```python
from build123d import *

# Parameters (mm, degrees)
F1_DEPTH = 10
F2_D     = 5.3
F4_D     = 4.2
F4_DEPTH = 10.4
F4_TIP   = 1.2618073


with BuildPart() as f1:
    # F0 (on Front) → F1 (new body)
    with BuildSketch(Plane.XZ):
        Polygon((35, -20), (35, 0), (35, 20), (-35, 20), (-35, -20), (-5.4585481157, -20), (-9.5, -27), (0, -27), (9.5, -27), (5.4585481157, -20), align=None)
    extrude(amount=-F1_DEPTH)

    # F2 (through all)
    with Locations(Plane.XZ):
        with Locations((0, 0)):
            Hole(F2_D / 2)

    # F4
    with Locations(Plane(origin=(0, 0, -20), x_dir=(1, 0, 0), z_dir=(0, 0, -1))):
        with Locations((-20, -5), (20, -5)):
            Hole(F4_D / 2, depth=F4_DEPTH)
            with Locations((0, 0, -(F4_DEPTH + F4_TIP / 2))):  # 118° drill point
                Cone(0, F4_D / 2, F4_TIP, mode=Mode.SUBTRACT)


solid = f1.part
```
Build history of the part. All positions in model axes, mm. A direction names the side the tool comes from. Round coordinates to 2 decimals unless told otherwise and drop trailing zeros. Loops run counter-clockwise (first coordinate to the right, second up) from the corner with the lowest first, then second, coordinate; pieces in that order, holes last.
Item 1: Drill centre lines: line 1 along Z through (x, y) = (0, 4.75); line 2 along X through (y, z) = (5.75, -15.5); line 3 along Y through (x, z) = (-20, -15). Where is each one in solid material? Low to high.
Item 2: Saw through at C-C (x = 0). List the corners of the cut face in (y, z), then the cut area to 3 significant figures.
Item 3: Two-plate mould, pull along Y, no slides. Class faces 1 (the face through (0, 0, -3)), 2 (the face through (-20.364, 4.984, -8.557)), 3 (the face through (0, 10, -3)), 4 (the face through (0, 5, 20)): released by +Y, released by -Y, zero draft, split by the parting line, or undercut.
Item 4: Saw through at D-D (z = -13.5). List the corners of the cut face in (x, y), then the cut area to 3 significant figures.
Item 5: Pin check, flat tip, straight feed: P1, Ø5, axis at x = -17.5, y = 3.5, coming from the -Z side. Stop position of the tip, or through.
Item 6: Saw through at B-B (y = 1.75). List the corners of the cut face in (x, z), then the cut area to 3 significant figures.
Item 7: Which spindle directions (+Z, -Z, +X, -X, +Y, -Y) get a long thin tool onto all of the face, cutting with end or side? Do faces 5 (the face through (-2.45, 5.07, -1.01)), 6 (the face through (7.51, 4.93, -23.55)), 7 (the face through (-7.45, 4.93, -23.45)), 8 (the face through (-21.94, 5.8, -14.73)). Say none if no direction does.
Item 8: Saw through at A-A (z = 0). List the corners of the cut face in (x, y).
Worked answers:
1. line 1: z = -27 to -2.65, 2.65 to 20
1. line 2: x = -35 to -21.96, -18.04 to 18.04, 21.96 to 35
1. line 3: y = 0 to 2.9, 7.1 to 10
2. outline: (0, -27) - (10, -27) - (10, -2.65) - (0, -2.65) - close; (0, 2.65) - (10, 2.65) - (10, 20) - (0, 20) - close
2. area: 417 mm2
3. face 1: released by -Y
3. face 2: undercut
3. face 3: released by +Y
3. face 4: zero draft
4. outline: (-35, 0) - (35, 0) - (35, 10) - (-35, 10) - close; hole circle Ø4.2 at (-20, 5); hole circle Ø4.2 at (20, 5)
4. area: 672 mm2
5. P1: stops at z = -20
6. outline: (-35, -20) - (-5.46, -20) - (-9.5, -27) - (9.5, -27) - (5.46, -20) - (35, -20) - (35, 20) - (-35, 20) - close; hole circle Ø5.3 at (0, 0)
6. area: 2,880 mm2
7. face 5: +Y, -Y
7. face 6: +X, +Y, -Y
7. face 7: -X, +Y, -Y
7. face 8: -Z
8. outline: (-35, 0) - (-2.65, 0) - (-2.65, 10) - (-35, 10) - close; (2.65, 0) - (35, 0) - (35, 10) - (2.65, 10) - close
